The listing builds one solid part. Answer for the finished solid, in the listing's coordinates (mm). Face numbers are marked on the shaded views. A direction names the side the tool comes from. Give positions to 0.01 mm unless a question says otherwise; leave off trailing zeros. Loops run counter-clockwise (first coordinate to the right, second up) from the corner with the lowest first, then second, coordinate; pieces in that order, holes last. Notation, with made-up numbers: (18.25, 20) - (43.25, 20) arc R23 cw to (43.25, 46) - close; hole circle Ø11 at (49.5, 30.25). An arc over 180 degrees is marked (long way). Write each question's results on one line, items separated by ' | '.
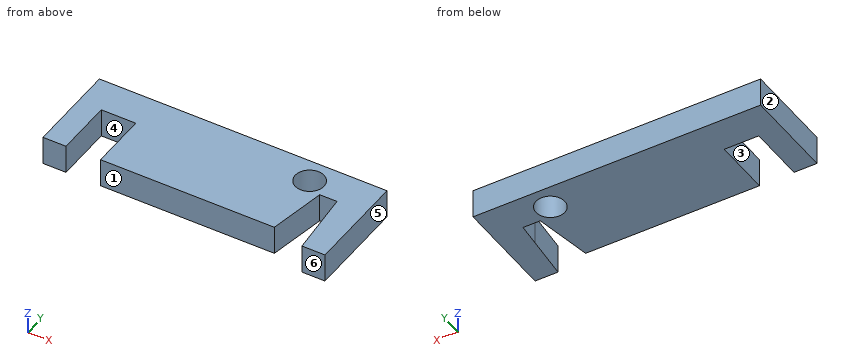
from build123d import *

# Parameters (mm, degrees)
SKETCH1_R           = 3.175
BOSS_EXTRUDE1_DEPTH = 3.175
SKETCH2_W           = 7.62
SKETCH2_H           = 12.7
CUT_EXTRUDE1_DEPTH  = 7.35


with BuildPart() as part:
    # Sketch1 → Boss-Extrude1 (new body, symmetric)
    with BuildSketch(Plane.XY):
        Polygon((21.571117009, -1.27), (25.381117009, -1.27), (25.82555942, -6.35), (31.75, -6.35), (31.75, 6.35), (0, 6.35), (-6.35, 6.35), (-31.75, 6.35), (-31.75, -6.35), (20.675375947, -6.35), align=None)
        with Locations((17.78, 1.27)):
            Circle(SKETCH1_R, mode=Mode.SUBTRACT)
        Polygon((19.331764354, -13.97), (20.675375947, -6.35), (-31.75, -6.35), (-31.75, -13.97), align=None)
        Polygon((31.75, -6.35), (25.82555942, -6.35), (26.67, -16.002), (31.75, -16.002), align=None)
    extrude(amount=BOSS_EXTRUDE1_DEPTH, both=True)

    # Sketch2 → Cut-Extrude1 (cut, through all)
    with BuildSketch(Plane.XY.offset(3.175)):
        with Locations((-22.86, -7.62)):
            Rectangle(SKETCH2_W, SKETCH2_H)
    extrude(amount=-CUT_EXTRUDE1_DEPTH, mode=Mode.SUBTRACT)


solid = part.part
Item 1: For a pull along X with two mould halves and no side action, classify the marked faces 4, 5 and 6 as released by +X, released by -X, zero draft, split by the parting line, or undercut.
Values found:
face 4: undercut | face 5: released by +X | face 6: zero draft
Item 2: Find the intervals of material crossed by line 1 along X through (y, z) = (-13, 1); line 2 along X through (y, z) = (-6.5, 0.25); line 3 along Y through (x, z) = (17.78, 1) (3 decimals), in increasing order. Write a range as [from, to].
Values found:
line 1: x = [-31.75, -26.67], [-19.05, 19.5], [26.41, 31.75] | line 2: x = [-31.75, -26.67], [-19.05, 20.65], [25.84, 31.75] | line 3: y = [-13.97, -1.905], [4.445, 6.35]
Item 3: A cutting plane is placed at A-A, the plane y = 1.27. Determine the outline of the cut face in (x, z) (3 decimals), plus the area to 3 significant figures.
Values found:
outline: (-31.75, -3.175) - (14.605, -3.175) - (14.605, 3.175) - (-31.75, 3.175) - close; (20.955, -3.175) - (31.75, -3.175) - (31.75, 3.175) - (20.955, 3.175) - close | area: 363 mm²
Item 4: A cutting plane is placed at D-D, the plane y = -9.25. Determine the outline of the cut face in (x, z) (3 decimals).
Values found:
outline: (-31.75, -3.175) - (-26.67, -3.175) - (-26.67, 3.175) - (-31.75, 3.175) - close; (-19.05, -3.175) - (20.164, -3.175) - (20.164, 3.175) - (-19.05, 3.175) - close; (26.079, -3.175) - (31.75, -3.175) - (31.75, 3.175) - (26.079, 3.175) - close
Item 5: A cutting plane is placed at C-C, the plane z = 0.75. Determine the outline of the cut face in (x, y) (3 decimals), plus the area to 3 significant figures.
Values found:
outline: (-31.75, -13.97) - (-26.67, -13.97) - (-26.67, -1.27) - (-19.05, -1.27) - (-19.05, -13.97) - (19.332, -13.97) - (21.571, -1.27) - (25.381, -1.27) - (26.67, -16.002) - (31.75, -16.002) - (31.75, 6.35) - (-31.75, 6.35) - close; hole circle Ø6.35 at (17.78, 1.27) | area: 1,100 mm²
Item 6: Flat-ended cylindrical pins translate along their axes: P1, Ø3, axis at x = -9.5, z = -0.5, coming from the -Y side; P2, Ø2, axis at x = -25.5, z = -1.5, coming from the -Y side; P3, Ø10, axis at x = 17.78, y = 1.27, coming from the +Z side (3 decimals). Find the tip coordinate at first contact, or state that the pin passes through.
Values found:
P1: stops at y = -13.97 | P2: stops at y = -1.27 | P3: stops at z = 3.175
Item 7: For the marked faces 1, 2 and 3, determine the directions among +Z, -Z, +X, -X, +Y, -Y from which every point of the face is accessible in a straight line to the end or side of a thin tool.
Values found:
face 1: +Z, -Z, -X, -Y | face 2: +Z, -Z, -X, +Y, -Y | face 3: +Z, -Z, -Y
Item 8: A cutting plane is placed at B-B, the plane x = 17.78. Determine the outline of the cut face in (y, z) (3 decimals), plus the area to 3 significant figures.
Values found:
outline: (-13.97, -3.175) - (-1.905, -3.175) - (-1.905, 3.175) - (-13.97, 3.175) - close; (4.445, -3.175) - (6.35, -3.175) - (6.35, 3.175) - (4.445, 3.175) - close | area: 88.7 mm²
